The drawing under review shows one solid part. Ordinate dimensions are in mm from its lowest x, y, z. A direction names the side the tool comes from. Coordinates: 2 decimals unless noted, no trailing zeros. Order: outer loops, then holes, each group sorted by start corner. A loop starts at its lowest first (then second) coordinate and runs counter-clockwise, first axis right, second up.
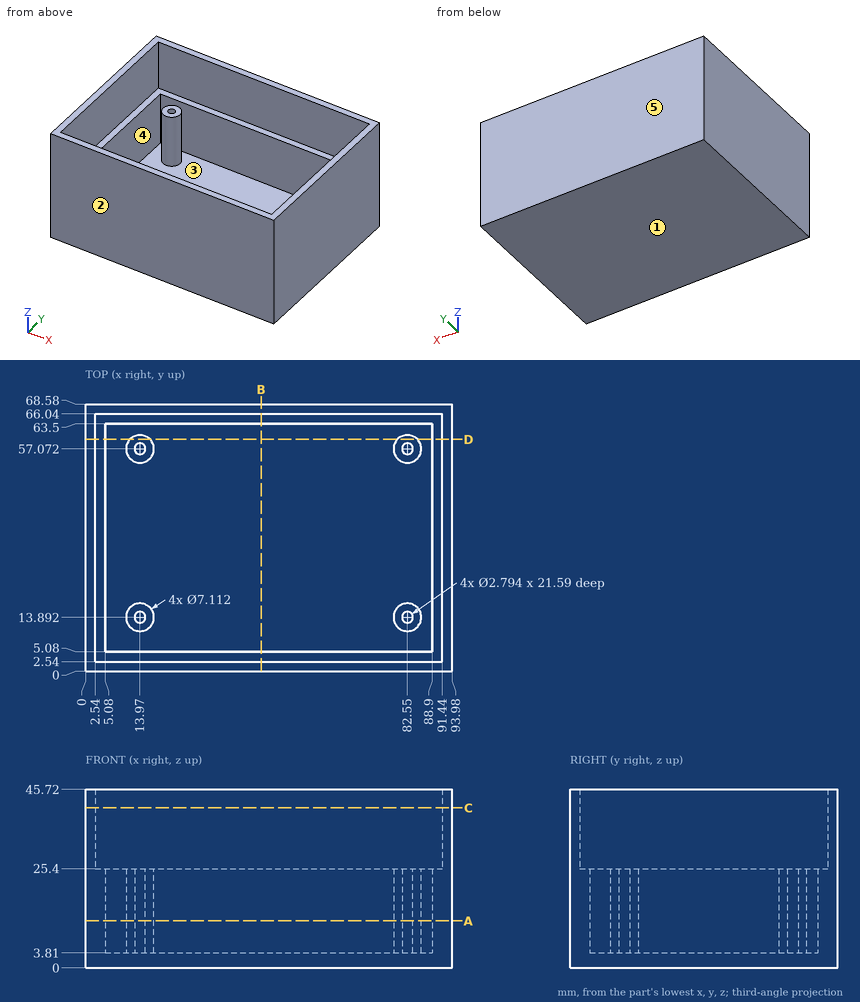
1. Take a section at C-C, the plane z = 41. Give the boundary of the cut face in (x, y).
Answer below:
outline: (0, 0) - (93.98, 0) - (93.98, 68.58) - (0, 68.58) - close; hole (2.54, 2.54) - (91.44, 2.54) - (91.44, 66.04) - (2.54, 66.04) - close
2. Machinability: for the marked faces 4 and 5, which of the approach directions +Z, -Z, +X, -X, +Y, -Y give a long, thin tool a straight path to every point of the face, cutting with its end or side? Answer none if there is none.
Answer below:
face 4: +Z
face 5: +Z, -Z, +X, -X, +Y
3. Take a section at A-A, the plane z = 12. Give the number of separate pieces and of enclosed holes in the cut face, plus the area to 3 significant figures.
Answer below:
separate pieces: 5
enclosed holes: 5
area: 1,680 mm2
4. To check wall thickness, follow L1, parallel to Y at x = 13.97, z = 19.5 (1 decimal); L2, parallel to X at y = 18, z = 20; L3, parallel to Y at x = 81, z = 14. State the ranges of each line that lie inside material, in increasing order.
Answer below:
L1: y = 0 to 5.1, 10.3 to 12.5, 15.3 to 17.4, 53.5 to 55.7, 58.5 to 60.6, 63.5 to 68.6
L2: x = 0 to 5.08, 88.9 to 93.98
L3: y = 0 to 5.08, 10.69 to 17.09, 53.87 to 60.27, 63.5 to 68.58
5. Take a section at D-D, the plane y = 59.5. Give the boundary of the cut face in (x, z).
Answer below:
outline: (0, 0) - (93.98, 0) - (93.98, 45.72) - (91.44, 45.72) - (91.44, 25.4) - (88.9, 25.4) - (88.9, 3.81) - (85.15, 3.81) - (85.15, 25.4) - (79.95, 25.4) - (79.95, 3.81) - (16.57, 3.81) - (16.57, 25.4) - (11.37, 25.4) - (11.37, 3.81) - (5.08, 3.81) - (5.08, 25.4) - (2.54, 25.4) - (2.54, 45.72) - (0, 45.72) - close
6. Clearance check with flat-ended pins moving along their axes: pin 1 Ø1 at (x, y) = (80, 60.5) entering from -Z; pin 2 Ø2 at (x, y) = (13.5, 14.5) entering from +Z; pin 3 Ø0.8 at (x, y) = (82.5, 13.5) entering from +Z. State where each tip first meets the part, or that it passes through.
Answer below:
pin 1: stops at z = 0
pin 2: stops at z = 25.4
pin 3: stops at z = 3.81
7. Take a section at B-B, the plane x = 45. Give the boundary of the cut face in (y, z).
Answer below:
outline: (0, 0) - (68.58, 0) - (68.58, 45.72) - (66.04, 45.72) - (66.04, 25.4) - (63.5, 25.4) - (63.5, 3.81) - (5.08, 3.81) - (5.08, 25.4) - (2.54, 25.4) - (2.54, 45.72) - (0, 45.72) - close
8. The part is to be moulded in two halves that separate along Y. For the marked faces 1, 2 and 3, say which applies: +Y half, -Y half, draft (parallel to the pull), parting line (faces both ways), or undercut.
Answer below:
face 1: draft
face 2: -Y half
face 3: undercut
